Read the model definition and answer for the solid it produces. Units are mm, in the model's axes. Face numbers are marked on the shaded views. A direction names the side the tool comes from. Coordinates: 2 decimals unless noted, no trailing zeros. Write each loop counter-clockwise with the first axis right and the second up, starting at its lowest first coordinate (ties: lowest second). Pieces come first, ordered by that corner, then holes. Notation, with made-up numbers: M 57,28.25 L 94,28.25 A20 ccw 94,38.25 Z; hole C 49.5,-21 d5. An arc over 180 degrees is marked long. Use a Markdown table: item, result. Add a question column.
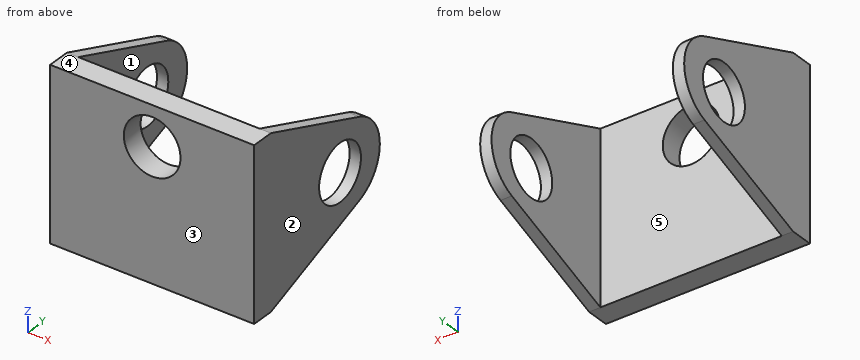
from build123d import *

# Parameters (mm, degrees)
SKETCH1_W               = 32
SKETCH1_H               = 4
BOSS_EXTRUDE1_DEPTH     = 30
CUT_EXTRUDE1_DEPTH      = 45.810713005
CUT_EXTRUDE1_DEPTH_BACK = 45.810713005
SKETCH2_R               = 5
CUT_EXTRUDE2_DEPTH      = 45.810713005
CUT_EXTRUDE2_DEPTH_BACK = 45.810713005
SKETCH3_R               = 5


with BuildPart() as part:
    # Sketch1 → Boss-Extrude1 (new body)
    with BuildSketch(Plane.XY):
        Polygon((-18, -2), (-16, -2), (-16, 2), (-16, 28), (-18, 28), align=None)
        Rectangle(SKETCH1_W, SKETCH1_H)
        Polygon((16, 2), (16, -2), (18, -2), (18, 28), (16, 28), align=None)
    extrude(amount=-BOSS_EXTRUDE1_DEPTH)

    # Sketch2 → Cut-Extrude1 (cut, two sides: drawn at the far end of the back side and taken through both)
    with BuildSketch(Plane(origin=(0, 0, 0), x_dir=(0, 0, -1), z_dir=(1, 0, 0)).offset(-CUT_EXTRUDE1_DEPTH_BACK)):
        with BuildLine():
            ThreePointArc((22.016723912, 23.148695064), (15, 28), (7.983276088, 23.148695064))
            Line((7.983276088, 23.148695064), (0, 2))
            Line((0, 2), (-5, 2))
            Line((-5, 2), (-5, 38))
            Line((-5, 38), (35, 38))
            Line((35, 38), (35, 2))
            Line((35, 2), (30, 2))
            Line((30, 2), (22.016723912, 23.148695064))
        make_face()
        with Locations((15, 18.5)):
            Circle(SKETCH2_R)
    extrude(amount=CUT_EXTRUDE1_DEPTH + CUT_EXTRUDE1_DEPTH_BACK, mode=Mode.SUBTRACT)

    # Sketch3 → Cut-Extrude2 (cut, two sides: drawn at the far end of the back side and taken through both)
    with BuildSketch(Plane(origin=(0, 0, 0), x_dir=(1, 0, 0), z_dir=(0, 1, 0)).offset(-CUT_EXTRUDE2_DEPTH_BACK)):
        with Locations(Location((0, 7, 0), (0, 0, 270))):
            Circle(SKETCH3_R)
    extrude(amount=CUT_EXTRUDE2_DEPTH + CUT_EXTRUDE2_DEPTH_BACK, mode=Mode.SUBTRACT)


solid = part.part
Item 1: Determine the mould class of the marked faces 1, 2 and 3 for opening direction X: pulls with the +X half, pulls with the -X half, needs draft (parallel to the pull), parting line crosses it, or undercut.
Item 2: Find section B-B on z = -15. Give the vertices of the cut face in (x, y).
Item 3: Find section D-D on y = 18.5. Give the vertices of the cut face in (x, z).
Item 4: Consider probe 1 along X at (y, z) = (10, -6); probe 2 along Z at (x, y) = (0, -0.5); probe 3 along Y at (x, z) = (2, -13.5). Determine where each line is inside the solid, lowest interval first.
Item 5: Find section A-A on x = 0. Give the vertices of the cut face in (y, z).
Item 6: For the marked faces 4 and 5, determine the directions among +Z, -Z, +X, -X, +Y, -Y from which every point of the face is accessible in a straight line to the end or side of a thin tool.
Item 7: Each of these flat-tipped pins is pushed along its axis until it touches: pin 1 (12 mm diameter, centred on x = 5, z = -5.5, fed in from +Y); pin 2 (8 mm diameter, centred on x = -12.5, z = -11, fed in from +Y). Where does it stop, or does it pass through?
Item 8: Find section C-C on y = 4. Give the vertices of the cut face in (x, z), then the cut area to 3 significant figures.
Geometry says:
| question | item | result |
|---|---|---|
| 1 | face 1 | undercut |
| 1 | face 2 | pulls with the +X half |
| 1 | face 3 | needs draft |
| 2 | outline | M -18,-2 L 18,-2 L 18,13.5 L 16,13.5 L 16,2 L -16,2 L -16,13.5 L -18,13.5 Z; M -18,23.5 L -16,23.5 L -16,28 L -18,28 Z; M 16,23.5 L 18,23.5 L 18,28 L 16,28 Z |
| 3 | outline | M -18,-23.77 L -16,-23.77 L -16,-20 L -18,-20 Z; M -18,-10 L -16,-10 L -16,-6.23 L -18,-6.23 Z; M 16,-23.77 L 18,-23.77 L 18,-20 L 16,-20 Z; M 16,-10 L 18,-10 L 18,-6.23 L 16,-6.23 Z |
| 4 | probe 1 | x = -18 to -16, 16 to 18 |
| 4 | probe 2 | z = -30 to -12, -2 to 0 |
| 4 | probe 3 | y = -2 to 2 |
| 5 | outline | M -2,-30 L 2,-30 L 2,-12 L -2,-12 Z; M -2,-2 L 2,-2 L 2,0 L -2,0 Z |
| 6 | face 4 | +Z, +X, -X, +Y, -Y |
| 6 | face 5 | +Z, -Z, +Y |
| 7 | pin 1 | stops at y = 2 |
| 7 | pin 2 | stops at y = 27.71 |
| 8 | outline | M -18,-29.25 L -16,-29.25 L -16,-0.75 L -18,-0.75 Z; M 16,-29.25 L 18,-29.25 L 18,-0.75 L 16,-0.75 Z |
| 8 | area | 114 mm2 |
